Could you check a few things on this model? Use its own coordinates, in mm. A direction names the side the tool comes from. Give positions to 0.01 mm unless a question says otherwise; leave off trailing zeros. Order: outer loops, then holes, each group sorted by start corner. A loop starts at its lowest first (then second) coordinate and runs counter-clockwise, first axis right, second up. Notation, with made-up numbers: (69.25, 4.25) - (76.25, 4.25) arc R24 ccw to (76.25, 37.25) - close; hole circle Ø5 at (80.25, 74). An arc over 180 degrees is marked (long way). Put each result on its own line as item: value.
from build123d import *

# Parameters (mm, degrees)
F0_W         = 279.4
F0_H         = 279.4
F0_W_2       = 266.7
F0_H_2       = 266.7
F0_W_3       = 254
F0_H_3       = 254
F0_W_4       = 241.3
F0_H_4       = 241.3
F1_DEPTH     = 6.35
F2_DEPTH     = 19.05
F3_SIZE      = 1.27
F4_R         = 2.54
F5_T1_DEPTH  = 274.32
F5_T3_DEPTH  = 274.32
F5_T5_DEPTH  = 13.97
F5_S9_W      = 2.54
F5_S9_H      = 2.54
F5_T10_DEPTH = 2.54
F5_S15_W     = 2.54
F5_S15_H     = 2.54
F5_T16_DEPTH = 2.54
F5_S21_W     = 2.54
F5_S21_H     = 2.54
F5_T22_DEPTH = 2.54
F5_S27_W     = 2.54
F5_S27_H     = 2.54
F5_T28_DEPTH = 2.54
F5_S33_W     = 2.54
F5_S33_H     = 2.54
F5_T34_DEPTH = 2.54
F5_S39_W     = 2.54
F5_S39_H     = 2.54
F5_T40_DEPTH = 2.54
F5_S45_W     = 2.54
F5_S45_H     = 2.54
F5_T46_DEPTH = 2.54
F5_S51_W     = 2.54
F5_S51_H     = 2.54
F5_T52_DEPTH = 2.54


# Not quite as in the source:
# - a fillet or chamfer that OpenCascade refuses, or shapes differently, is made with other operations: its cross-section is extruded or revolved along the edge and cut away or added


with BuildPart() as f1:
    # F0 (on Top) → F1 (new body)
    with BuildSketch(Plane.XY):
        Rectangle(F0_W, F0_H)
        Rectangle(F0_W_2, F0_H_2, mode=Mode.SUBTRACT)
        Rectangle(F0_W_2, F0_H_2)
        Rectangle(F0_W_3, F0_H_3, mode=Mode.SUBTRACT)
        Rectangle(F0_W_3, F0_H_3)
        Rectangle(F0_W_4, F0_H_4, mode=Mode.SUBTRACT)
        Rectangle(F0_W_4, F0_H_4)
    extrude(amount=F1_DEPTH)

    # F0 (on Top) → F2 (join)
    with BuildSketch(Plane.XY):
        Rectangle(F0_W, F0_H)
        Rectangle(F0_W_2, F0_H_2, mode=Mode.SUBTRACT)
        Rectangle(F0_W_3, F0_H_3)
        Rectangle(F0_W_4, F0_H_4, mode=Mode.SUBTRACT)
    extrude(amount=F2_DEPTH)

    # F3
    f3_edges = [f1.edges().sort_by_distance(p)[0] for p in [
        (-127, 0, 19.05),
        (-133.35, 0, 19.05),
        (0, 133.35, 19.05),
        (0, 127, 19.05),
        (133.35, 0, 19.05),
        (127, 0, 19.05),
        (0, -127, 19.05),
        (0, -133.35, 19.05),
    ]]
    chamfer(f3_edges, length=F3_SIZE)

    # F4
    f4_edges = [f1.edges().sort_by_distance(p)[0] for p in [
        (-139.7, 0, 19.05),
        (0, 139.7, 19.05),
        (139.7, 0, 19.05),
        (0, -139.7, 19.05),
        (-120.65, 0, 19.05),
        (0, -120.65, 19.05),
        (120.65, 0, 19.05),
        (0, 120.65, 19.05),
    ]]
    fillet(f4_edges, radius=F4_R)

    # F5: fillet of radius 2.54 on 8 edges, made by hand

    # F5_s2 → F5_t1 (cut)
    with BuildSketch(Plane.YZ.offset(-137.16)):
        with BuildLine():
            ThreePointArc((139.7, 2.54), (138.9560512242, 0.7439487758), (137.16, 0))
            Line((137.16, 0), (139.7, 0))
            Line((139.7, 0), (139.7, 2.54))
        make_face()
        with BuildLine():
            ThreePointArc((-139.7, 2.54), (-138.9560512242, 0.7439487758), (-137.16, 0))
            Line((-137.16, 0), (-139.7, 0))
            Line((-139.7, 0), (-139.7, 2.54))
        make_face()
    extrude(amount=F5_T1_DEPTH, mode=Mode.SUBTRACT)

    # F5_s4 → F5_t3 (cut)
    with BuildSketch(Plane.XZ.offset(-137.16)):
        with BuildLine():
            ThreePointArc((-139.7, 2.54), (-138.9560512242, 0.7439487758), (-137.16, 0))
            Line((-137.16, 0), (-139.7, 0))
            Line((-139.7, 0), (-139.7, 2.54))
        make_face()
        with BuildLine():
            ThreePointArc((139.7, 2.54), (138.9560512242, 0.7439487758), (137.16, 0))
            Line((137.16, 0), (139.7, 0))
            Line((139.7, 0), (139.7, 2.54))
        make_face()
    extrude(amount=F5_T3_DEPTH, mode=Mode.SUBTRACT)

    # F5_s6 → F5_t5 (cut)
    with BuildSketch(Plane.XY.offset(2.54)):
        with BuildLine():
            ThreePointArc((137.16, 139.7), (138.9560512242, 138.9560512242), (139.7, 137.16))
            Line((139.7, 137.16), (139.7, 139.7))
            Line((139.7, 139.7), (137.16, 139.7))
        make_face()
        with BuildLine():
            ThreePointArc((-139.7, 137.16), (-138.9560512242, 138.9560512242), (-137.16, 139.7))
            Line((-137.16, 139.7), (-139.7, 139.7))
            Line((-139.7, 139.7), (-139.7, 137.16))
        make_face()
        with BuildLine():
            ThreePointArc((-139.7, -137.16), (-138.9560512242, -138.9560512242), (-137.16, -139.7))
            Line((-137.16, -139.7), (-139.7, -139.7))
            Line((-139.7, -139.7), (-139.7, -137.16))
        make_face()
        with BuildLine():
            ThreePointArc((137.16, -139.7), (138.9560512242, -138.9560512242), (139.7, -137.16))
            Line((139.7, -137.16), (139.7, -139.7))
            Line((139.7, -139.7), (137.16, -139.7))
        make_face()
    extrude(amount=F5_T5_DEPTH, mode=Mode.SUBTRACT)


with BuildPart() as f5_tool8:
    # F5_s9 → F5_t10 (new body)
    with BuildSketch(Plane.XZ.offset(137.16)):
        with Locations((138.43, 17.78)):
            Rectangle(F5_S9_W, F5_S9_H)
    extrude(amount=F5_T10_DEPTH)

    # F5_s11 → F5_t12 (revolve, cut)
    with BuildSketch(Plane(origin=(137.16, -137.16, 16.51), x_dir=(-0.7071067812, 0, -0.7071067812), z_dir=(-0.7071067812, 0, 0.7071067812))):
        with BuildLine():
            ThreePointArc((0, -2.54), (2.54, 0), (0, 2.54))
            Line((0, 2.54), (0, -2.54))
        make_face()
    revolve(axis=Axis((137.16, -137.16, 16.51), (0, -1, 0)), mode=Mode.SUBTRACT)


with BuildPart() as f1_1:
    add(f1.part)

    # F5_t7: cut F5_tool8
    add(f5_tool8.part, mode=Mode.SUBTRACT)


with BuildPart() as f5_tool14:
    # F5_s15 → F5_t16 (new body)
    with BuildSketch(Plane.YZ.offset(-137.16)):
        with Locations((-138.43, 17.78)):
            Rectangle(F5_S15_W, F5_S15_H)
    extrude(amount=-F5_T16_DEPTH)

    # F5_s17 → F5_t18 (revolve, cut)
    with BuildSketch(Plane(origin=(-137.16, -137.16, 16.51), x_dir=(0, 0.7071067812, -0.7071067812), z_dir=(0, 0.7071067812, 0.7071067812))):
        with BuildLine():
            ThreePointArc((0, -2.54), (2.54, 0), (0, 2.54))
            Line((0, 2.54), (0, -2.54))
        make_face()
    revolve(axis=Axis((-137.16, -137.16, 16.51), (-1, 0, 0)), mode=Mode.SUBTRACT)


with BuildPart() as f1_2:
    add(f1_1.part)

    # F5_t13: cut F5_tool14
    add(f5_tool14.part, mode=Mode.SUBTRACT)


with BuildPart() as f5_tool20:
    # F5_s21 → F5_t22 (new body)
    with BuildSketch(Plane.YZ.offset(-137.16)):
        with Locations((138.43, 17.78)):
            Rectangle(F5_S21_W, F5_S21_H)
    extrude(amount=-F5_T22_DEPTH)

    # F5_s23 → F5_t24 (revolve, cut)
    with BuildSketch(Plane(origin=(-137.16, 137.16, 16.51), x_dir=(0, -0.7071067812, -0.7071067812), z_dir=(0, 0.7071067812, -0.7071067812))):
        with BuildLine():
            ThreePointArc((0, -2.54), (2.54, 0), (0, 2.54))
            Line((0, 2.54), (0, -2.54))
        make_face()
    revolve(axis=Axis((-137.16, 137.16, 16.51), (-1, 0, 0)), mode=Mode.SUBTRACT)


with BuildPart() as f1_3:
    add(f1_2.part)

    # F5_t19: cut F5_tool20
    add(f5_tool20.part, mode=Mode.SUBTRACT)


with BuildPart() as f5_tool26:
    # F5_s27 → F5_t28 (new body)
    with BuildSketch(Plane.XZ.offset(-137.16)):
        with Locations((138.43, 17.78)):
            Rectangle(F5_S27_W, F5_S27_H)
    extrude(amount=-F5_T28_DEPTH)

    # F5_s29 → F5_t30 (revolve, cut)
    with BuildSketch(Plane(origin=(137.16, 137.16, 16.51), x_dir=(-0.7071067812, 0, -0.7071067812), z_dir=(0.7071067812, 0, -0.7071067812))):
        with BuildLine():
            ThreePointArc((0, -2.54), (2.54, 0), (0, 2.54))
            Line((0, 2.54), (0, -2.54))
        make_face()
    revolve(axis=Axis((137.16, 137.16, 16.51), (0, 1, 0)), mode=Mode.SUBTRACT)


with BuildPart() as f1_4:
    add(f1_3.part)

    # F5_t25: cut F5_tool26
    add(f5_tool26.part, mode=Mode.SUBTRACT)


with BuildPart() as f5_tool32:
    # F5_s33 → F5_t34 (new body)
    with BuildSketch(Plane.XY.offset(2.54)):
        with Locations((138.43, 138.43)):
            Rectangle(F5_S33_W, F5_S33_H)
    extrude(amount=-F5_T34_DEPTH)

    # F5_s35 → F5_t36 (revolve, cut)
    with BuildSketch(Plane(origin=(137.16, 137.16, 2.54), x_dir=(-0.7071067812, -0.7071067812, 0), z_dir=(0.7071067812, -0.7071067812, 0))):
        with BuildLine():
            ThreePointArc((0, -2.54), (2.54, 0), (0, 2.54))
            Line((0, 2.54), (0, -2.54))
        make_face()
    revolve(axis=Axis((137.16, 137.16, 2.54), (0, 0, -1)), mode=Mode.SUBTRACT)


with BuildPart() as f1_5:
    add(f1_4.part)

    # F5_t31: cut F5_tool32
    add(f5_tool32.part, mode=Mode.SUBTRACT)


with BuildPart() as f5_tool38:
    # F5_s39 → F5_t40 (new body)
    with BuildSketch(Plane.XY.offset(2.54)):
        with Locations((-138.43, 138.43)):
            Rectangle(F5_S39_W, F5_S39_H)
    extrude(amount=-F5_T40_DEPTH)

    # F5_s41 → F5_t42 (revolve, cut)
    with BuildSketch(Plane(origin=(-137.16, 137.16, 2.54), x_dir=(0.7071067812, -0.7071067812, 0), z_dir=(0.7071067812, 0.7071067812, 0))):
        with BuildLine():
            ThreePointArc((0, -2.54), (2.54, 0), (0, 2.54))
            Line((0, 2.54), (0, -2.54))
        make_face()
    revolve(axis=Axis((-137.16, 137.16, 2.54), (0, 0, -1)), mode=Mode.SUBTRACT)


with BuildPart() as f1_6:
    add(f1_5.part)

    # F5_t37: cut F5_tool38
    add(f5_tool38.part, mode=Mode.SUBTRACT)


with BuildPart() as f5_tool44:
    # F5_s45 → F5_t46 (new body)
    with BuildSketch(Plane.YZ.offset(-137.16)):
        with Locations((-138.43, 1.27)):
            Rectangle(F5_S45_W, F5_S45_H)
    extrude(amount=-F5_T46_DEPTH)

    # F5_s47 → F5_t48 (revolve, cut)
    with BuildSketch(Plane(origin=(-137.16, -137.16, 2.54), x_dir=(0, 0.7071067812, 0.7071067812), z_dir=(0, -0.7071067812, 0.7071067812))):
        with BuildLine():
            ThreePointArc((0, -2.54), (2.54, 0), (0, 2.54))
            Line((0, 2.54), (0, -2.54))
        make_face()
    revolve(axis=Axis((-137.16, -137.16, 2.54), (-1, 0, 0)), mode=Mode.SUBTRACT)


with BuildPart() as f1_7:
    add(f1_6.part)

    # F5_t43: cut F5_tool44
    add(f5_tool44.part, mode=Mode.SUBTRACT)


with BuildPart() as f5_tool50:
    # F5_s51 → F5_t52 (new body)
    with BuildSketch(Plane.XY.offset(2.54)):
        with Locations((138.43, -138.43)):
            Rectangle(F5_S51_W, F5_S51_H)
    extrude(amount=-F5_T52_DEPTH)

    # F5_s53 → F5_t54 (revolve, cut)
    with BuildSketch(Plane(origin=(137.16, -137.16, 2.54), x_dir=(-0.7071067812, 0.7071067812, 0), z_dir=(-0.7071067812, -0.7071067812, 0))):
        with BuildLine():
            ThreePointArc((0, -2.54), (2.54, 0), (0, 2.54))
            Line((0, 2.54), (0, -2.54))
        make_face()
    revolve(axis=Axis((137.16, -137.16, 2.54), (0, 0, -1)), mode=Mode.SUBTRACT)


with BuildPart() as f1_8:
    add(f1_7.part)

    # F5_t49: cut F5_tool50
    add(f5_tool50.part, mode=Mode.SUBTRACT)


solid = f1_8.part
1) If I drill on line 1 (X direction, y = 6.5, z = 13.5); line 2 (Y direction, x = 122.5, z = 8.5), over which ranges is the centre line in solid material (lowest first)? Write a range as [from, to].
Filled in:
line 1: x = [-139.7, -133.35], [-127, -120.65], [120.65, 127], [133.35, 139.7]
line 2: y = [-139.7, -133.35], [-127, 127], [133.35, 139.7]
2) We'd pull the mould along X, two halves only. Please class faces 1 (the flat face through (139.7, -2, 9)), 2 (the flat face through (-2, 139.7, 9)), 3 (the flat face through (127, -2, 12)): pulls with the +X half, pulls with the -X half, needs draft (parallel to the pull), parting line crosses it, or undercut.
Filled in:
face 1: pulls with the +X half
face 2: needs draft
face 3: undercut
3) I'm going to push a flat-ended pin straight in: pin 1 (3 mm diameter, centred on x = -85.5, y = -10, fed in from +Z). Where does the tip first touch, or does it pass through?
Filled in:
pin 1: stops at z = 6.35
4) Suppose I cut it at A-A, the plane z = 10.25. List the corners of the cut face in (x, y) for me.
Filled in:
outline: (-139.7, -137.16) arc R2.54 ccw to (-137.16, -139.7) - (137.16, -139.7) arc R2.54 ccw to (139.7, -137.16) - (139.7, 137.16) arc R2.54 ccw to (137.16, 139.7) - (-137.16, 139.7) arc R2.54 ccw to (-139.7, 137.16) - close; (-127, -127) - (127, -127) - (127, 127) - (-127, 127) - close; hole (-133.35, -133.35) - (133.35, -133.35) - (133.35, 133.35) - (-133.35, 133.35) - close; hole (-120.65, -120.65) - (120.65, -120.65) - (120.65, 120.65) - (-120.65, 120.65) - close
5) Suppose I cut it at B-B, the plane x = -66. List the corners of the cut face in (y, z) for me, and give its area (3 significant figures).
Filled in:
outline: (-139.7, 2.54) arc R2.54 ccw to (-137.16, 0) - (137.16, 0) arc R2.54 ccw to (139.7, 2.54) - (139.7, 16.51) arc R2.54 ccw to (137.16, 19.05) - (134.62, 19.05) - (133.35, 17.78) - (133.35, 6.35) - (127, 6.35) - (127, 17.78) - (125.73, 19.05) - (123.19, 19.05) arc R2.54 ccw to (120.65, 16.51) - (120.65, 6.35) - (-120.65, 6.35) - (-120.65, 16.51) arc R2.54 ccw to (-123.19, 19.05) - (-125.73, 19.05) - (-127, 17.78) - (-127, 6.35) - (-133.35, 6.35) - (-133.35, 17.78) - (-134.62, 19.05) - (-137.16, 19.05) arc R2.54 ccw to (-139.7, 16.51) - close
area: 2,090 mm^2
6) Which directions (+Z, -Z, +X, -X, +Y, -Y) give clear straight access to the entire face, cutting with the end or side of a thin tool? Please do faces 4 (the flat face through (-120.65, -2, 11)), 5 (the flat face through (-2, 2, 0)).
Filled in:
face 4: +Z
face 5: -Z, +X, -X, +Y, -Y
